from build123d import *

# Parameters (mm, degrees)
SKETCH1_W           = 275
SKETCH1_H           = 100
BOSS_EXTRUDE4_DEPTH = 4.75
SKETCH3_R           = 1.5
SKETCH3_W           = 60
SKETCH3_H           = 12.5
CUT_EXTRUDE1_DEPTH  = 10
SKETCH4_R           = 1.85
SKETCH4_R_2         = 1.375
CUT_EXTRUDE2_DEPTH  = 10


with BuildPart() as part:
    # Sketch1 → Boss-Extrude4 (new body)
    with BuildSketch(Plane(origin=(0, 0, 0), x_dir=(1, 0, 0), z_dir=(0, 1, 0))):
        Rectangle(SKETCH1_W, SKETCH1_H)
    extrude(amount=BOSS_EXTRUDE4_DEPTH)

    # Sketch3 → Cut-Extrude1 (cut)
    with BuildSketch(Plane(origin=(0, 4.75, 0), x_dir=(1, 0, 0), z_dir=(0, 1, 0))):
        with Locations(Location((119.3, -30, 0), (0, 0, 270))):
            Circle(SKETCH3_R)
        with Locations(Location((119.3, 30, 0), (0, 0, 270))):
            Circle(SKETCH3_R)
        with Locations((107.5, -43.75)):
            Rectangle(SKETCH3_W, SKETCH3_H)
        with Locations((107.5, 43.75)):
            Rectangle(SKETCH3_W, SKETCH3_H)
        with BuildLine():
            Line((2.5, -50), (-57.5, -50))
            Line((-57.5, -50), (-57.5, -37.5))
            ThreePointArc((-57.5, -37.5), (-55.690778624, -27.2393957), (-50.481333294, -18.216371709))
            Line((-50.481333294, -18.216371709), (-4.518666706, -18.216371709))
            ThreePointArc((-4.518666706, -18.216371709), (0.690778624, -27.2393957), (2.5, -37.5))
            Line((2.5, -37.5), (2.5, -50))
        make_face()
        with BuildLine():
            Line((2.5, 50), (-57.5, 50))
            Line((-57.5, 50), (-57.5, 37.5))
            ThreePointArc((-57.5, 37.5), (-55.690778624, 27.2393957), (-50.481333294, 18.216371709))
            Line((-50.481333294, 18.216371709), (-4.518666706, 18.216371709))
            ThreePointArc((-4.518666706, 18.216371709), (0.690778624, 27.2393957), (2.5, 37.5))
            Line((2.5, 37.5), (2.5, 50))
        make_face()
    extrude(amount=-CUT_EXTRUDE1_DEPTH, mode=Mode.SUBTRACT)

    # Sketch4 → Cut-Extrude2 (cut)
    with BuildSketch(Plane(origin=(0, 4.75, 0), x_dir=(1, 0, 0), z_dir=(0, 1, 0))):
        with Locations(Location((-127.5, -26.25, 0), (0, 0, 270))):
            Circle(SKETCH4_R)
        with Locations(Location((-114.8, -26.25, 0), (0, 0, 270))):
            Circle(SKETCH4_R)
        with Locations(Location((-127.5, -8.75, 0), (0, 0, 270))):
            Circle(SKETCH4_R)
        with Locations(Location((-114.8, -8.75, 0), (0, 0, 270))):
            Circle(SKETCH4_R)
        with Locations(Location((-114.8, 8.75, 0), (0, 0, 270))):
            Circle(SKETCH4_R)
        with Locations(Location((-127.5, 8.75, 0), (0, 0, 270))):
            Circle(SKETCH4_R)
        with Locations(Location((-114.8, 26.25, 0), (0, 0, 270))):
            Circle(SKETCH4_R)
        with Locations(Location((-127.5, 26.25, 0), (0, 0, 270))):
            Circle(SKETCH4_R)
        with Locations(Location((71.25, -43.75, 0), (0, 0, 270))):
            Circle(SKETCH4_R_2)
        with Locations(Location((22.25, -43.75, 0), (0, 0, 270))):
            Circle(SKETCH4_R_2)
        with Locations(Location((71.25, 14.25, 0), (0, 0, 270))):
            Circle(SKETCH4_R_2)
        with Locations(Location((22.25, 14.25, 0), (0, 0, 270))):
            Circle(SKETCH4_R_2)
    extrude(amount=-CUT_EXTRUDE2_DEPTH, mode=Mode.SUBTRACT)


solid = part.part
Geometry check sheet. Reference: the model listing, model coordinates, mm. A direction names the side the tool comes from. Round coordinates to 2 decimals unless told otherwise and drop trailing zeros. Order: outer loops, then holes, each group sorted by start corner. A loop starts at its lowest first (then second) coordinate and runs counter-clockwise, first axis right, second up. Notation, with made-up numbers: M 27.5,7.5 L 35.5,7.5 A20 cw 35.5,13.5 Z; hole C 60.25,-37 d9. An arc over 180 degrees is marked long. Answer in a Markdown table with one row per item. Add a question column.
Item 1: Material ranges on L1, parallel to X at y = 2.7, z = -8.75; L2, parallel to Z at x = 119.3, y = 3.65; L3, parallel to Z at x = 71.25, y = 3.65 (3 decimals), recorded low to high. Write a range as [from, to].
Item 2: Sectioned sample at A-A, the plane z = -43. Enter the section's corners in (x, y), plus the area to 3 significant figures.
Item 3: Sectioned sample at B-B, the plane y = 0.9. State how many separate pieces and enclosed holes the cut face has, plus the area to 3 significant figures.
Item 4: Set-up check for faces 5 (the face through (-28, 2, -18.216)), 6 (the face through (107, 2, -37.5)), 7 (the face through (-57.5, 2, 44)), 8 (the face through (77.5, 2, 44)): record each of +Z, -Z, +X, -X, +Y, -Y from which the full face is reachable in a straight line by a thin tool's end or side.
Item 5: Depth check by flat-ended pin: pin 1 Ø1.4 at (y, z) = (3.5, 44.5) entering from +X. Enter the tip coordinate at first touch or a pass-through.
Item 6: Draft check along X on faces 1 (the face through (39, 2, 50)), 2 (the face through (-137.5, 2, 1)), 3 (the face through (0.64, 2.41, 27.1)), 4 (the face through (2.5, 2, 44)). Enter one of: released by +X, released by -X, zero draft, split by the parting line, or undercut.
Filled in:
| question | item | result |
|---|---|---|
| 1 | L1 | x = [-137.5, -129.35], [-125.65, -116.65], [-112.95, 137.5] |
| 1 | L2 | z = [-37.5, -31.5], [-28.5, 28.5], [31.5, 37.5] |
| 1 | L3 | z = [-50, -15.625], [-12.875, 42.375], [45.125, 50] |
| 2 | outline | M -137.5,0 L -57.5,0 L -57.5,4.75 L -137.5,4.75 Z; M 2.5,0 L 77.5,0 L 77.5,4.75 L 2.5,4.75 Z |
| 2 | area | 736 mm² |
| 3 | separate pieces | 1 |
| 3 | enclosed holes | 14 |
| 3 | area | 22,200 mm² |
| 4 | face 5 | -Z, +Y, -Y |
| 4 | face 6 | -Z, +X, +Y, -Y |
| 4 | face 7 | +Z, +Y, -Y |
| 4 | face 8 | +Z, +X, +Y, -Y |
| 5 | pin 1 | stops at x = 77.5 |
| 6 | face 1 | zero draft |
| 6 | face 2 | released by -X |
| 6 | face 3 | undercut |
| 6 | face 4 | undercut |
